Read the model definition and answer for the solid it produces. Units are mm, in the model's axes. Give positions to 0.01 mm unless a question says otherwise; leave off trailing zeros. Order: outer loops, then holes, each group sorted by start corner. A loop starts at its lowest first (then second) coordinate and runs counter-clockwise, first axis right, second up.
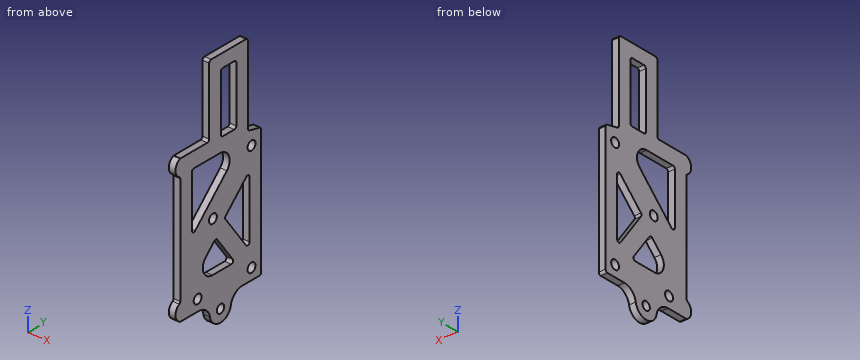
```python
from build123d import *

# Parameters (mm, degrees)
SKETCH_1_R          = 2.05
SKETCH_1_R_2        = 1.9
EXTRUDE_1_DEPTH     = 3
SKETCH_2_W          = 27
SKETCH_2_H          = 8
CUT_EXTRUDE_1_DEPTH = 3
FILLET_1_R          = 5
FILLET_2_R          = 1
FILLET_3_R          = 6


with BuildPart() as part:
    # 草图1 → 凸台-拉伸1 (new body)
    with BuildSketch(Plane(origin=(0, 0, 0), x_dir=(0, 0, -1), z_dir=(1, 0, 0))):
        with BuildLine():
            Line((29.1, -22.95), (29.1, -7.630182627))
            Line((29.1, -7.630182627), (33.194571076, -7.630182627))
            ThreePointArc((33.194571076, -7.630182627), (38.694571076, -2.130182627), (33.194571076, 3.369817373))
            Line((33.194571076, 3.369817373), (29.1, 3.369817373))
            Line((29.1, 3.369817373), (29.1, 18.95))
            Line((29.1, 18.95), (-29.1, 18.95))
            Line((-29.1, 18.95), (-30.699580381, 12.05))
            Line((-30.699580381, 12.05), (-67.336045252, 12.05))
            Line((-67.336045252, 12.05), (-67.336045252, -7.95))
            Line((-67.336045252, -7.95), (-35.336045252, -7.95))
            Line((-35.336045252, -7.95), (-35.336045252, -22.95))
            ThreePointArc((-35.336045252, -22.95), (-31.627946009, -25.45), (-27.919846765, -22.95))
            Line((-27.919846765, -22.95), (21.683801513, -22.95))
            ThreePointArc((21.683801513, -22.95), (25.391900756, -25.45), (29.1, -22.95))
        make_face()
        with Locations((-24.1, 13.95)):
            Circle(SKETCH_1_R, mode=Mode.SUBTRACT)
        with Locations((24.1, 13.95)):
            Circle(SKETCH_1_R, mode=Mode.SUBTRACT)
        with Locations((24.1, -13.95)):
            Circle(SKETCH_1_R, mode=Mode.SUBTRACT)
        with Locations((-4.1, -6.05)):
            Circle(SKETCH_1_R, mode=Mode.SUBTRACT)
        with Locations((33.194571076, -2.130182627)):
            Circle(SKETCH_1_R_2, mode=Mode.SUBTRACT)
    extrude(amount=EXTRUDE_1_DEPTH)

    # 草图2 → 切除-拉伸1 (cut)
    with BuildSketch(Plane(origin=(3, 0, 0), x_dir=(0, 0, -1), z_dir=(1, 0, 0))):
        Polygon((-28.336045252, 9.700763878), (-28.336045252, -16.95), (-1.685281374, -16.95), align=None)
        with Locations((-47.836045252, 2.05)):
            Rectangle(SKETCH_2_W, SKETCH_2_H)
        Polygon((18.1, 5.403799603), (4.202253287, -4.45275835), (18.1, -18.350505063), align=None)
        Polygon((-14.614718626, 12.95), (16.63985744, 12.95), (-1.646014864, -0.018703762), align=None)
    extrude(amount=-CUT_EXTRUDE_1_DEPTH, mode=Mode.SUBTRACT)

    # 圆角1
    fillet_1_edges = [part.edges().sort_by_distance(p)[0] for p in [
        (1.5, -18.350505063, -18.1),
        (1.5, 9.700763878, 28.336045252),
    ]]
    fillet(fillet_1_edges, radius=FILLET_1_R)

    # 圆角2
    fillet_2_edges = [part.edges().sort_by_distance(p)[0] for p in [
        (1.5, 18.95, 29.1),
        (1.5, 18.95, -29.1),
        (1.5, -22.95, -21.683801513),
        (1.5, -22.95, 27.919846765),
        (1.5, -7.95, 35.336045252),
        (1.5, -7.95, 67.336045252),
        (1.5, 12.05, 67.336045252),
        (1.5, 12.05, 30.699580381),
        (1.5, -1.95, 61.336045252),
        (1.5, 6.05, 61.336045252),
        (1.5, 6.05, 34.336045252),
        (1.5, -1.95, 34.336045252),
        (1.5, -0.018703762, 1.646014864),
        (1.5, 12.95, 14.614718626),
        (1.5, 12.95, -16.63985744),
        (1.5, 5.403799603, -18.1),
        (1.5, -4.45275835, -4.202253287),
        (1.5, -16.95, 1.685281374),
        (1.5, -16.95, 28.336045252),
    ]]
    fillet(fillet_2_edges, radius=FILLET_2_R)

    # 圆角3
    fillet_3_edges = [part.edges().sort_by_distance(p)[0] for p in [
        (1.5, -7.630182627, -29.1),
        (1.5, 3.369817373, -29.1),
    ]]
    fillet(fillet_3_edges, radius=FILLET_3_R)


solid = part.part
```
1) The part is cut by section B-B on y = 13.95. Determine the outline of the cut face in (x, z).
Final values:
outline: (0, -29.1) - (3, -29.1) - (3, -26.15) - (0, -26.15) - close; (0, -22.05) - (3, -22.05) - (3, 22.05) - (0, 22.05) - close; (0, 26.15) - (3, 26.15) - (3, 30.26) - (0, 30.26) - close
2) Given pin 1 (1.5 mm diameter, centred on x = 1, y = -11.5, fed in from -Z); pin 2 (1.5 mm diameter, centred on x = 1, z = 14, fed in from -Y); pin 3 (1.5 mm diameter, centred on x = 2, z = 54.5, fed in from -Y), each flat-ended and moving along its own axis, determine where each tip first touches the part or whether it passes through.
Final values:
pin 1: stops at z = -29.75
pin 2: stops at y = -22.95
pin 3: stops at y = -7.95
3) Consider L1, parallel to Y at x = 0.8, z = 0; L2, parallel to Y at x = 2.35, z = -8.5; L3, parallel to Z at x = 2.2, y = -8.5. Determine where each line is inside the solid, lowest interval first.
Final values:
L1: y = -22.95 to 1.15, 12.95 to 18.95
L2: y = -22.95 to -8.75, -1.4 to 7.18, 12.95 to 18.95
L3: z = -31.74 to -17.58, -8.25 to 10.14, 28.34 to 35.44
4) The part is cut by section A-A on z = -24.1. Determine the outline of the cut face in (x, y), and give its area (3 significant figures).
Final values:
outline: (0, -25.24) - (3, -25.24) - (3, -16) - (0, -16) - close; (0, -11.9) - (3, -11.9) - (3, 11.9) - (0, 11.9) - close; (0, 16) - (3, 16) - (3, 18.95) - (0, 18.95) - close
area: 108 mm2
5) The part is cut by section D-D on z = -3.5. Determine the outline of the cut face in (x, y), and give its area (3 significant figures).
Final values:
outline: (0, -22.95) - (3, -22.95) - (3, 3.63) - (0, 3.63) - close; (0, 12.95) - (3, 12.95) - (3, 18.95) - (0, 18.95) - close
area: 97.7 mm2
6) The part is cut by section C-C on z = 47. Determine the outline of the cut face in (x, y), and give its area (3 significant figures).
Final values:
outline: (0, -7.95) - (3, -7.95) - (3, -1.95) - (0, -1.95) - close; (0, 6.05) - (3, 6.05) - (3, 12.05) - (0, 12.05) - close
area: 36.0 mm2
